Could you check a few things on this model? Use its own coordinates, in mm. A direction names the side the tool comes from. Give positions to 0.01 mm unless a question says otherwise; leave off trailing zeros. Write each question's results on one line, items separated by ' | '. Start each with the question number.
Q1. We'd pull the mould along Z, two halves only. Please class faces 3 (the face through (13, 217, 8)), 4 (the face through (8, 217, 1.5)), 5 (the face through (8, 217, 13)), 6 (the face through (10, 0, 12)): released by +Z, released by -Z, zero draft, split by the parting line, or undercut.
Q2. Will these pins go through, and if not, where does the flat tip stop? P1, Ø1.4, axis at y = 256.5, z = 21.5, coming from the +X side; P2, Ø7, axis at x = 7, y = 195, coming from the +Z side; P3, Ø0.5, axis at x = 21.5, y = 172.5, coming from the -Z side.
Q3. Which directions (+Z, -Z, +X, -X, +Y, -Y) give clear straight access to the entire face, cutting with the end or side of a thin tool? Please do faces 1 (the face through (17, 217, 23)), 2 (the face through (1.5, 217, 8)).
Q4. If I drill on line 1 along X through (y, z) = (176, 17); line 2 along Z through (x, y) = (8, 405.5); line 3 along X through (y, z) = (294.5, 8.25), over which ranges is the centre line in solid material (lowest first)?
Q5. If we section it at A-A, the plane y = 338: Give the number of separate pieces and of enclosed holes in the cut face, plus the area to 3 significant figures.
from build123d import *

# Parameters (mm, degrees)
AUFSATZ_LINEAR_AUSTRAGEN1_DEPTH = 440


with BuildPart() as part:
    # Skizze1 → Aufsatz-Linear austragen1 (new body)
    with BuildSketch(Plane.XZ):
        with BuildLine():
            Line((3.450001515, 23.00000001), (2.5, 23.00000001))
            ThreePointArc((2.5, 23.00000001), (0.73223304, 22.26776696), (-1e-08, 20.5))
            Line((-1e-08, 20.5), (-1e-08, 2.50000002))
            ThreePointArc((-1e-08, 2.50000002), (0.732233039, 0.732233062), (2.499999998, 1.2e-08))
            Line((2.499999998, 1.2e-08), (20.499999977, 1.2e-08))
            ThreePointArc((20.499999977, 1.2e-08), (22.267766938, 0.732233062), (22.999999988, 2.500000023))
            Line((22.999999988, 2.500000023), (22.999999988, 3.450004181))
            ThreePointArc((22.999999988, 3.450004181), (22.912132793, 3.662134355), (22.700002619, 3.75000155))
            Line((22.700002619, 3.75000155), (20.999999992, 3.75000155))
            ThreePointArc((20.999999992, 3.75000155), (20.6464466, 3.60355494), (20.49999999, 3.250001548))
            Line((20.49999999, 3.250001548), (20.49999999, 1.500001969))
            ThreePointArc((20.49999999, 1.500001969), (20.412132795, 1.287871795), (20.200002621, 1.2000046))
            Line((20.200002621, 1.2000046), (15.86065559, 1.2000046))
            Line((15.86065559, 1.2000046), (12.99999999, 4.0606602))
            Line((12.99999999, 4.0606602), (12.99999999, 11.93933984))
            Line((12.99999999, 11.93933984), (15.86065559, 14.79999544))
            Line((15.86065559, 14.79999544), (20.200002638, 14.79999544))
            ThreePointArc((20.200002638, 14.79999544), (20.4121328, 14.71212825), (20.49999999, 14.499998088))
            Line((20.49999999, 14.499998088), (20.49999999, 12.749998492))
            ThreePointArc((20.49999999, 12.749998492), (20.6464466, 12.3964451), (20.999999992, 12.24999849))
            Line((20.999999992, 12.24999849), (22.700002636, 12.24999849))
            ThreePointArc((22.700002636, 12.24999849), (22.912132798, 12.33786568), (22.999999988, 12.549995842))
            Line((22.999999988, 12.549995842), (22.999999988, 20.5))
            ThreePointArc((22.999999988, 20.5), (22.267766938, 22.26776696), (20.499999977, 23.00000001))
            Line((20.499999977, 23.00000001), (12.549998485, 23.00000001))
            ThreePointArc((12.549998485, 23.00000001), (12.33786644, 22.91213204), (12.24999847, 22.699999995))
            Line((12.24999847, 22.699999995), (12.24999847, 21.000000012))
            ThreePointArc((12.24999847, 21.000000012), (12.39644508, 20.64644662), (12.749998472, 20.50000001))
            Line((12.749998472, 20.50000001), (14.499998051, 20.50000001))
            ThreePointArc((14.499998051, 20.50000001), (14.712128225, 20.412132815), (14.79999542, 20.200002641))
            Line((14.79999542, 20.200002641), (14.79999542, 15.86065561))
            Line((14.79999542, 15.86065561), (11.93933982, 13.00000001))
            Line((11.93933982, 13.00000001), (4.06066018, 13.00000001))
            Line((4.06066018, 13.00000001), (1.20000458, 15.86065561))
            Line((1.20000458, 15.86065561), (1.20000458, 20.200002658))
            ThreePointArc((1.20000458, 20.200002658), (1.28787177, 20.41213282), (1.500001932, 20.50000001))
            Line((1.500001932, 20.50000001), (3.250001528, 20.50000001))
            ThreePointArc((3.250001528, 20.50000001), (3.60355492, 20.64644662), (3.75000153, 21.000000012))
            Line((3.75000153, 21.000000012), (3.75000153, 22.699999995))
            ThreePointArc((3.75000153, 22.699999995), (3.66213356, 22.91213204), (3.450001515, 23.00000001))
        make_face()
        with BuildLine():
            Line((1.49999999, 3.767766952), (1.49999999, 12.715075784))
            ThreePointArc((1.49999999, 12.715075784), (1.685194957, 12.992239639), (2.012132015, 12.927207815))
            Line((2.012132015, 12.927207815), (3.146446603, 11.792893227))
            ThreePointArc((3.146446603, 11.792893227), (3.470869961, 11.57612047), (3.853553404, 11.5))
            Line((3.853553404, 11.5), (5.91421356, 11.5))
            Line((5.91421356, 11.5), (5.994865994, 11.419347566))
            ThreePointArc((5.994865994, 11.419347566), (6.158199998, 11.33547495), (6.339812993, 11.362481111))
            ThreePointArc((6.339812993, 11.362481111), (7.999999982, 11.750000011), (9.660186973, 11.362481114))
            ThreePointArc((9.660186973, 11.362481114), (9.841799967, 11.335474953), (10.00513397, 11.419347568))
            Line((10.00513397, 11.419347568), (10.085786402, 11.5))
            Line((10.085786402, 11.5), (10.999999968, 11.5))
            ThreePointArc((10.999999968, 11.5), (11.35355336, 11.35355339), (11.49999997, 10.999999998))
            Line((11.49999997, 10.999999998), (11.49999997, 10.085786456))
            Line((11.49999997, 10.085786456), (11.41934753, 10.005134016))
            ThreePointArc((11.41934753, 10.005134016), (11.335474915, 9.841800012), (11.362481077, 9.660187017))
            ThreePointArc((11.362481077, 9.660187017), (11.749999981, 8.00000002), (11.362481081, 6.339813023))
            ThreePointArc((11.362481081, 6.339813023), (11.33547492, 6.158200028), (11.419347536, 5.994866024))
            Line((11.419347536, 5.994866024), (11.49999997, 5.91421359))
            Line((11.49999997, 5.91421359), (11.49999997, 3.853553434))
            ThreePointArc((11.49999997, 3.853553434), (11.57612044, 3.470869991), (11.792893197, 3.146446633))
            Line((11.792893197, 3.146446633), (12.927207774, 2.012132056))
            ThreePointArc((12.927207774, 2.012132056), (12.992239599, 1.685194995), (12.715075743, 1.500000027))
            Line((12.715075743, 1.500000027), (3.767766925, 1.500000027))
            ThreePointArc((3.767766925, 1.500000027), (3.305827172, 1.808658302), (3.414213544, 2.353553394))
            Line((3.414213544, 2.353553394), (4.41421357, 3.35355342))
            ThreePointArc((4.41421357, 3.35355342), (4.576425223, 3.461939781), (4.767766914, 3.50000001))
            Line((4.767766914, 3.50000001), (6.563859334, 3.50000001))
            ThreePointArc((6.563859334, 3.50000001), (7.05645152, 3.91425072), (6.732817059, 4.47058825))
            ThreePointArc((6.732817059, 4.47058825), (5.348349567, 5.348349579), (4.470588229, 6.732817064))
            ThreePointArc((4.470588229, 6.732817064), (3.914250698, 7.056451522), (3.49999999, 6.563859337))
            Line((3.49999999, 6.563859337), (3.49999999, 4.767766934))
            ThreePointArc((3.49999999, 4.767766934), (3.461939761, 4.576425243), (3.3535534, 4.41421359))
            Line((3.3535534, 4.41421359), (2.353553374, 3.414213564))
            ThreePointArc((2.353553374, 3.414213564), (1.808658272, 3.305827189), (1.49999999, 3.767766952))
        make_face(mode=Mode.SUBTRACT)
        with BuildLine():
            Line((15.79999543, 17.299995436), (15.79999543, 21.499999998))
            ThreePointArc((15.79999543, 21.499999998), (15.94644204, 21.85355339), (16.299995432, 22))
            Line((16.299995432, 22), (20.499999977, 22))
            ThreePointArc((20.499999977, 22), (21.560660149, 21.560660172), (21.999999978, 20.5))
            Line((21.999999978, 20.5), (21.999999978, 16.299995432))
            ThreePointArc((21.999999978, 16.299995432), (21.853553368, 15.94644204), (21.499999976, 15.79999543))
            Line((21.499999976, 15.79999543), (17.299995436, 15.79999543))
            ThreePointArc((17.299995436, 15.79999543), (16.23933526, 16.23933526), (15.79999543, 17.299995436))
        make_face(mode=Mode.SUBTRACT)
    extrude(amount=-AUFSATZ_LINEAR_AUSTRAGEN1_DEPTH)


solid = part.part
Final values:
1) face 3: undercut | face 4: undercut | face 5: released by +Z | face 6: zero draft
2) P1: stops at x = 22.98 | P2: stops at z = 23 | P3: stops at z = 0.12
3) face 1: +Z, +X, -X, +Y, -Y | face 2: +Y, -Y
4) line 1: x = 0 to 1.2, 14.8 to 15.83, 22 to 23 | line 2: z = 0 to 1.5, 11.75 to 13 | line 3: x = 0 to 1.5, 11.74 to 13
5) separate pieces: 1 | enclosed holes: 2 | area: 164 mm²
